Geometry: final body of the model. Coordinates: model frame, mm. Round coordinates to 2 decimals unless told otherwise and drop trailing zeros. Write each loop counter-clockwise with the first axis right and the second up, starting at its lowest first coordinate (ties: lowest second). Pieces come first, ordered by that corner, then holes. Notation, with made-up numbers: M 88.25,6 L 147.25,6 A20 cw 147.25,30 Z; hole C 16.25,16.25 d11. An arc over 180 degrees is marked long. Put each result on its own line as item: value. Start each with the question number.
Autodesk Inventor part; units mm, degrees
ref_plane "YZ Plane" through (0, 0, 0) normal (1, 0, 0) x (0, 1, 0)
ref_plane "XZ Plane" through (0, 0, 0) normal (0, 1, 0) x (-1, 0, 0)
ref_plane "XY Plane" through (0, 0, 0) normal (0, 0, 1) x (1, 0, 0)
sketch "Sketch9" plane through (0, 0, 0) normal (0, 1, 0) x (-1, 0, 0)
  line L0 (0, 0) -> (-53.213, 0)
  line L1 (-53.213, 0) -> (-53.213, 36.3728)
  line L2 (0, 0) -> (0, 15.24)
  line L3 (0, 15.24) -> (-28.0555, 72.2061)
  arc A0 (-28.0555, 72.2061) -> (-53.213, 36.3728) centre (-16.1162, 37.0761) ccw
  dimension "d113" = 53.213
  dimension "d114" = 36.3728
  dimension "d115" = 15.24
  dimension "d116" = 63.5
  dimension "d117" = 153.78
extrude "Extrusion10" add sketch "Sketch9" along normal blind 1.5875
sketch "Sketch10" plane through (0, 1.5875, 0) normal (0, 1, 0) x (1, 0, 0)
  line L0 (53.213, -36.3728) -> (53.213, 0)
  line L1 (53.213, 0) -> (44.2468, 0)
  line L2 (53.213, 0) -> (0, 0)
  line L3 (44.2468, 0) -> (44.2468, -16.7386)
  line L4 (44.2468, 0) -> (44.2468, -42.1386)
  circle A0 centre (44.2468, -42.1386) radius 2.1844
  line L5 (44.2468, -42.1386) -> (31.5468, -42.1386)
  circle A1 centre (31.5468, -42.1386) radius 2.1844
  line L6 (53.213, 0) -> (27.813, 0)
  line L7 (31.5468, -42.1386) -> (31.5468, 0)
  line L8 (31.5468, -42.1386) -> (31.5468, -63.0936)
  circle A2 centre (31.5468, -63.0936) radius 2.1844
  circle A3 centre (42.0624, -54.2817) radius 2.1844
  arc A4 (31.5468, -63.0936) -> (44.2468, -42.1386) centre (25.3391, -45.0054) ccw
  line L9 (31.5468, 0) -> (31.5468, -16.7386)
  circle A5 centre (31.5468, -16.7386) radius 2.1844
  dimension "d123" = 8.9662
  dimension "d124" = 16.7386
  dimension "d126" = 42.1386
  dimension "d127" = 12.7
  dimension "d128" = 4.3688
  dimension "d129" = 25.4
  dimension "d130" = 20.955
  dimension "d131" = 4.3688
  dimension "d134" = 4.3688
  dimension "d142" = 16.7386
  dimension "d143" = 4.3688
fillet "Fillet4" radius 3.175 2 edges at (28.0555, 0.7937, 72.2061) (53.213, 0.7937, 0)
fillet "Fillet5" radius 3.175 1 edges at (0, 0.7937, 0)
fillet "Fillet6" radius 12.7 1 edges at (0, 0.7937, 15.24)
sketch "Sketch12" plane through (0, 1.5875, 0) normal (0, 1, 0) x (1, 0, 0)
  point P0 (0, 0)
  point P1 (3.175, 0)
extrude "Extrusion13" cut sketch "Sketch10" against normal blind 1.5875 contours A5 L7 | L7 A5 | A0 A4 L4 | L4 L5 A0 | A4 A0 L5 | L7 L8 A1 | A1 L5 L7 | A1 L8 L5 | A4 A3 | A3 A4 | A2 A4 L8 | L8 A4 A2
properties part number "New-Sleds" material "Polycarbonate, Clear"
1) Ray query, probe 1 along X at (y, z) = (1.4, 5.5); probe 2 along X at (y, z) = (0.95, 56); probe 3 along Z at (x, y) = (44.5, 0.8). Return the intervals inside material, ascending.
2) Section C-C, the plane y = 0.3. Output: boundary loops of the cut face in (x, z) (3 decimals).
3) Section D-D, the plane z = 64. Output: boundary loops of the cut face in (x, y), and give its area (3 significant figures).
4) First-contact query: pin 1 (12 mm diameter, centred on x = 47, z = 19, fed in from -Y). Flat tip, straight axial feed; report the tip coordinate or a pass-through.
5) Section B-B, the plane x = 32.5. Output: boundary loops of the cut face in (y, z), and give its area (3 significant figures).
6) Draft query along X for faces 1 (the face through (28.5, 0.8, 71.17)), 2 (the face through (29.94, 0.8, 15.26)), 3 (the face through (29.365, 0.805, 62.998)), 4 (the face through (27, 1.588, 28)). Return one class per face: +X half, -X half, draft (parallel to the pull), parting line (faces both ways), or undercut.
7) Section A-A, the plane z = 55. Output: boundary loops of the cut face in (x, y).
Solved:
1. probe 1: x = 0 to 53.21
1. probe 2: x = 20.07 to 40.71, 43.41 to 48.03
1. probe 3: z = 0 to 39.97, 44.31 to 60.97
2. outline: M 0,3.175 A3.175 ccw 3.175,0 L 50.038,0 A3.175 ccw 53.213,3.175 L 53.213,36.373 A37.104 ccw 30.886,71.113 A3.175 ccw 26.774,69.603 L 1.307,17.893 A12.7 ccw 0,12.282 Z; hole C 31.547,16.739 d4.369; hole C 31.547,42.139 d4.369; hole C 31.547,63.094 d4.369; hole C 42.062,54.282 d4.369; hole C 44.247,42.139 d4.369
3. outline: M 24.01,0 L 29.56,0 L 29.56,1.59 L 24.01,1.59 Z; M 33.53,0 L 41.65,0 L 41.65,1.59 L 33.53,1.59 Z
3. area: 21.7 mm2
4. pin 1: stops at y = 0
5. outline: M 0,0 L 1.59,0 L 1.59,14.77 L 0,14.77 Z; M 0,18.7 L 1.59,18.7 L 1.59,40.17 L 0,40.17 Z; M 0,44.1 L 1.59,44.1 L 1.59,61.13 L 0,61.13 Z; M 0,65.06 L 1.59,65.06 L 1.59,70.37 L 0,70.37 Z
5. area: 93.0 mm2
6. face 1: parting line
6. face 2: undercut
6. face 3: undercut
6. face 4: draft
7. outline: M 19.58,0 L 40,0 L 40,1.59 L 19.58,1.59 Z; M 44.13,0 L 48.6,0 L 48.6,1.59 L 44.13,1.59 Z
